from build123d import *

# Parameters (mm, degrees)
F0_R     = 38.1
F1_DEPTH = 76.2
F2_W     = 140.091866
F2_H     = 113.32272
F3_DEPTH = 25.4
F4_R     = 6.35


with BuildPart() as f1:
    # F0 (on Top) → F1 (new body)
    with BuildSketch(Plane.XY):
        Circle(F0_R)
    extrude(amount=F1_DEPTH)

    # F2 (on Top) → F3 (join)
    with BuildSketch(Plane.XY):
        Rectangle(F2_W, F2_H)
    extrude(amount=F3_DEPTH)

    # F4
    f4_edges = [f1.edges().sort_by_distance(p)[0] for p in [
        (-38.1, 0, 25.4),
    ]]
    fillet(f4_edges, radius=F4_R)


solid = f1.part
Input: part model. Units: mm. Frame: model coordinates. A direction names the side the tool comes from. Give positions to 0.01 mm unless a question says otherwise; leave off trailing zeros. Order: outer loops, then holes, each group sorted by start corner. A loop starts at its lowest first (then second) coordinate and runs counter-clockwise, first axis right, second up.
Q1. Section B-B on x = 0. Output: boundary loops of the cut face in (y, z), and give its area (3 significant figures).
Checked values:
outline: (-56.66, 0) - (56.66, 0) - (56.66, 25.4) - (44.45, 25.4) arc R6.35 cw to (38.1, 31.75) - (38.1, 76.2) - (-38.1, 76.2) - (-38.1, 31.75) arc R6.35 cw to (-44.45, 25.4) - (-56.66, 25.4) - close
area: 6,770 mm2
Q2. Ray query, probe 1 along Z at (x, y) = (-33, 29.5); probe 2 along Y at (x, z) = (-5, 31.5); probe 3 along X at (y, z) = (23, 69). Return the intervals inside material, ascending.
Checked values:
probe 1: z = 0 to 25.4
probe 2: y = -37.78 to 37.78
probe 3: x = -30.37 to 30.37
Q3. Set-up query: faces 1 (the flat face through (-1, -56.661, 13)), 2 (the cylindrical face through (-30.235, -23.183, 53.664)). Return all of +Z, -Z, +X, -X, +Y, -Y with unobstructed straight access to the full face (end or side cutting, diameter ignored); none if empty.
Checked values:
face 1: +Z, -Z, +X, -X, -Y
face 2: +Z
Q4. Section D-D on z = 30. Output: boundary loops of the cut face in (x, y).
Checked values:
outline: circle Ø76.69 at (0, 0)
Q5. Section C-C on z = 47. Output: boundary loops of the cut face in (x, y).
Checked values:
outline: circle Ø76.2 at (0, 0)
Q6. Section A-A on y = 0. Output: boundary loops of the cut face in (x, z).
Checked values:
outline: (-70.05, 0) - (70.05, 0) - (70.05, 25.4) - (44.45, 25.4) arc R6.35 cw to (38.1, 31.75) - (38.1, 76.2) - (-38.1, 76.2) - (-38.1, 31.75) arc R6.35 cw to (-44.45, 25.4) - (-70.05, 25.4) - close
Q7. Contact query for flat-ended pins moving along their axis: pin 1 Ø10 at (y, z) = (-37.5, 52.5) entering from +X; pin 2 Ø1 at (x, z) = (-22, 57) entering from -Y; pin 3 Ø1 at (y, z) = (27, 50) entering from +X. Output: stop coordinate, or through.
Checked values:
pin 1: stops at x = 19.88
pin 2: stops at y = -31.45
pin 3: stops at x = 27.37
